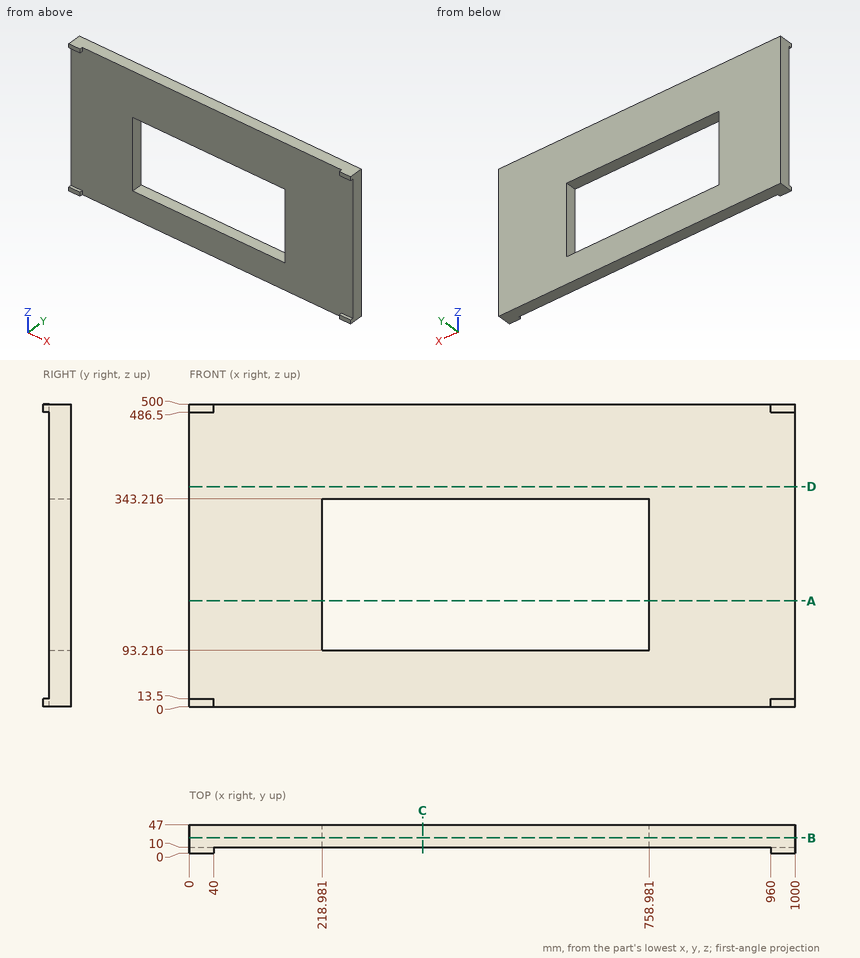
Study the drawing (mm; zero at the part's minimum x, y, z) and answer. Give positions to 0.01 mm unless a question says otherwise; leave off trailing zeros. Order: outer loops, then holes, each group sorted by start corner. A loop starts at its lowest first (then second) coordinate and runs counter-clockwise, first axis right, second up. Notation, with made-up numbers: (52.5, 47) - (102.5, 47) arc R28 ccw to (102.5, 76) - close; hole circle Ø4 at (57.5, 21.25). An arc over 180 degrees is marked (long way). Answer in a Markdown table with one row per item. Add a question column.
Q1. The part is cut by section C-C (x = 385). Determine the outline of the cut face in (y, z), then the cut area to 3 significant figures.
Q2. Given P1, Ø10, axis at x = 314.5, z = 433, coming from the -Y side, flat-ended and moving along its own axis, determine where the tip first touches the part or whether it passes through.
Q3. The part is cut by section D-D (z = 363.5). Determine the outline of the cut face in (x, y), then the cut area to 3 significant figures.
Q4. The part is cut by section A-A (z = 175). Determine the outline of the cut face in (x, y), then the cut area to 3 significant figures.
Q5. The part is cut by section B-B (y = 25.5). Determine the outline of the cut face in (x, z).
Q6. Find the intervals of material crossed by line 1 along X through (y, z) = (43, 206); line 2 along Z through (x, y) = (537, 22); line 3 along Y through (x, z) = (939, 191), in increasing order. Write a range as [from, to].
Determined:
| question | item | result |
|---|---|---|
| 1 | outline | (10, 0) - (47, 0) - (47, 93.22) - (10, 93.22) - close; (10, 343.22) - (47, 343.22) - (47, 500) - (10, 500) - close |
| 1 | area | 9,250 mm² |
| 2 | P1 | stops at y = 10 |
| 3 | outline | (0, 10) - (1000, 10) - (1000, 47) - (0, 47) - close |
| 3 | area | 37,000 mm² |
| 4 | outline | (0, 10) - (218.98, 10) - (218.98, 47) - (0, 47) - close; (758.98, 10) - (1000, 10) - (1000, 47) - (758.98, 47) - close |
| 4 | area | 17,000 mm² |
| 5 | outline | (0, 0) - (1000, 0) - (1000, 500) - (0, 500) - close; hole (218.98, 93.22) - (758.98, 93.22) - (758.98, 343.22) - (218.98, 343.22) - close |
| 6 | line 1 | x = [0, 218.98], [758.98, 1000] |
| 6 | line 2 | z = [0, 93.22], [343.22, 500] |
| 6 | line 3 | y = [10, 47] |
